Autodesk Inventor part; units mm, degrees
ref_plane "YZ Plane" through (0, 0, 0) normal (1, 0, 0) x (0, 1, 0)
ref_plane "XZ Plane" through (0, 0, 0) normal (0, 1, 0) x (-1, 0, 0)
ref_plane "XY Plane" through (0, 0, 0) normal (0, 0, 1) x (1, 0, 0)
sketch "Sketch1" plane through (0, 0, 0) normal (0, 0, 1) x (1, 0, 0)
  circle A0 centre (0, 0) radius 12.5 construction
  arc A1 (-7.8805, 17.3436) -> (7.8805, 17.3436) centre (0, 12.5) ccw
  arc A2 (-11.0798, -15.4965) -> (-18.9602, -1.8471) centre (-10.8253, -6.25) ccw
  arc A3 (18.9602, -1.8471) -> (11.0798, -15.4965) centre (10.8253, -6.25) ccw
  arc A4 (-7.8805, 17.3436) -> (-18.9602, -1.8471) centre (0, 0) ccw
  arc A5 (-11.0798, -15.4965) -> (11.0798, -15.4965) centre (0, 0) ccw
  arc A6 (18.9602, -1.8471) -> (7.8805, 17.3436) centre (0, 0) ccw
  dimension "d0" = 25
  dimension "d1" = 18.5
  dimension "d5" = 360
extrude "Extrusion1" add sketch "Sketch1" along normal blind 6.35
fillet "Fillet1" radius 0.762 6 edges at (-7.8805, 17.3436, 3.175) (7.8805, 17.3436, 3.175) (18.9602, -1.8471, 3.175) (11.0798, -15.4965, 3.175) (-11.0798, -15.4965, 3.175) (-18.9602, -1.8471, 3.175)
sketch "Sketch2" plane through (0, 0, 6.35) normal (0, 0, 1) x (1, 0, 0)
  circle A0 centre (0, 0) radius 14.9225 construction
  circle A1 centre (0, -14.9225) radius 2.5
  circle A2 centre (12.9233, 7.4612) radius 2.5
  circle A3 centre (-12.9233, 7.4613) radius 2.5
  dimension "d10" = 29.845
  dimension "d11" = 5
  dimension "d14" = 360
extrude "Extrusion2" cut sketch "Sketch2" against normal blind 6.35
sketch "Sketch3" plane through (0, 0, 6.35) normal (0, 0, 1) x (1, 0, 0)
  circle A0 centre (0, 0) radius 2.25
  dimension "d18" = 4.5
extrude "Extrusion3" cut sketch "Sketch3" against normal blind 6.35
properties part number "battery_holder"
The model under review builds one solid part; all positions refer to its coordinate system, in mm. Round coordinates to 2 decimals unless told otherwise and drop trailing zeros. Write each loop counter-clockwise with the first axis right and the second up, starting at its lowest first coordinate (ties: lowest second). Pieces come first, ordered by that corner, then holes.
(1) We need section B-B on y = 12.5. Give the boundary of the cut face in (x, z).
(2) We need section C-C on x = -8. Give the boundary of the cut face in (y, z), and give its area (3 significant figures).
(3) Mouldability with a two-part tool opening along X and no side actions: class faces 1 (the cylindrical face through (-16.564, 9.409, 3.131)), 2 (the cylindrical face through (-0.542, -17.363, 3.219)), 3 (the cylindrical face through (16.43, 9.64, 3.13)), 4 (the flat face through (0, -3, 0)) as +X half, -X half, draft (parallel to the pull), parting line (faces both ways), or undercut.
(4) We need section A-A on x = 0. Give the boundary of the cut face in (y, z), and give its area (3 significant figures).
(5) Wall thickness on L1, parallel to X at y = 9, z = 3; L2, parallel to X at y = -13, z = 3.5; L3, parallel to X at y = 2, z = 0.75: over which ranges is each line inside the solid? List them lowest first.
(6) Insertion check: pin 1 (2 mm diameter, centred on y = -15, z = 3, fed in from -X); pin 2 (11 mm diameter, centred on x = 10.83, y = -6.25, fed in from +Z); pin 3 (2 mm diameter, centred on y = 9, z = 5.5, fed in from -X); pin 4 (2 mm diameter, centred on x = -2, z = 4.5, fed in from -Y). Each pin has a flat end and moves straight along its axis. Give the tip position at first contact, or say it passes through.
(7) We need section D-D on z = 5.75. Give the number of separate pieces and of enclosed holes in the cut face, and give its area (3 significant figures).
Findings below:
1. outline: (-14.38, 0) - (-9.25, 0) - (-9.25, 6.35) - (-14.38, 6.35) - close; (9.25, 0) - (14.38, 0) - (14.38, 6.35) - (9.25, 6.35) - close
2. outline: (-17.29, 0) - (-15.06, 0) - (-15.06, 6.35) - (-17.29, 6.35) - close; (2.56, 0) - (7.86, 0) - (7.86, 6.35) - (2.56, 6.35) - close
2. area: 47.8 mm2
3. face 1: -X half
3. face 2: undercut
3. face 3: +X half
3. face 4: draft
4. outline: (-19.05, 0) - (-17.42, 0) - (-17.42, 6.35) - (-19.05, 6.35) - close; (-12.42, 0) - (-2.25, 0) - (-2.25, 6.35) - (-12.42, 6.35) - close; (2.25, 0) - (3.25, 0) - (3.25, 6.35) - (2.25, 6.35) - close
4. area: 81.3 mm2
5. L1: x = -16.79 to -14.89, -10.95 to -8.56, 8.56 to 10.95, 14.89 to 16.79
5. L2: x = -4.5 to -1.6, 1.6 to 4.5
5. L3: x = -18.94 to -15.01, -6.64 to -1.03, 1.03 to 6.64, 15.01 to 18.94
6. pin 1: stops at x = -9.53
6. pin 2: passes through
6. pin 3: stops at x = -17.29
6. pin 4: stops at y = -19.02
7. separate pieces: 1
7. enclosed holes: 4
7. area: 346 mm2
